Can you work these out from the model? Positions are in its coordinate system, mm. A direction names the side the tool comes from. Coordinates: 2 decimals unless noted, no trailing zeros. Write each loop counter-clockwise with the first axis right and the second up, starting at its lowest first coordinate (ties: lowest second). Pieces come first, ordered by that corner, then holes. Notation, with made-up numbers: (42.5, 34) -> (65.5, 34) arc R26 ccw to (65.5, 71) -> close; hole circle Ø10 at (54.5, 16). An arc over 180 degrees is marked (long way). Answer as CSV lines item,"result". Start each with the question number.
Autodesk Inventor part; units mm, degrees
ref_plane "YZ Plane" through (0, 0, 0) normal (1, 0, 0) x (0, 1, 0)
ref_plane "XZ Plane" through (0, 0, 0) normal (0, 1, 0) x (-1, 0, 0)
ref_plane "XY Plane" through (0, 0, 0) normal (0, 0, 1) x (1, 0, 0)
sketch "Sketch1" plane through (0, 0, 0) normal (0, 0, 1) x (1, 0, 0)
  line L0 (-19.313, 5.3077) -> (234.687, 5.3077)
  line L1 (234.687, 5.3077) -> (234.687, 0.3077)
  line L2 (234.687, 0.3077) -> (-19.313, 0.3077)
  line L3 (-19.313, 0.3077) -> (-19.313, 5.3077)
  line L4 (44.187, 5.3077) -> (44.187, 0.3077) construction
  line L5 (171.187, 5.3077) -> (171.187, 0.3077) construction
  line L6 (107.687, 5.3077) -> (107.687, 0.3077) construction
  point P0 (0, 0)
  dimension "d0" = 254
  dimension "d1" = 5
  dimension "d2" = 63.5
  dimension "d3" = 63.5
  dimension "d4" = 63.5
extrude "Extrusion1" add sketch "Sketch1" along normal blind 5
sketch "Sketch2" plane through (0, 0, 0) normal (0, 0, -1) x (-1, 0, 0)
  line L0 (19.313, 0.3077) -> (-234.687, 0.3077)
  arc A0 (-20.4966, 0.3077) -> (-14.937, 4.3077) centre (-20.4966, 6.1713) ccw
  arc A1 (-9.937, 4.3077) -> (-4.3774, 0.3077) centre (-4.3774, 6.1713) ccw
  line L1 (-14.937, 4.3077) -> (-9.937, 4.3077)
  line L2 (19.313, 0.3077) -> (-234.687, 0.3077)
  line L3 (-234.687, 5.3077) -> (19.313, 5.3077)
  arc A2 (-82.7042, 0.3077) -> (-78.437, 3.8077) centre (-82.7042, 4.659) ccw
  arc A3 (-73.437, 3.8077) -> (-69.1698, 0.3077) centre (-69.1698, 4.659) ccw
  line L4 (-78.437, 3.8077) -> (-73.437, 3.8077)
  arc A4 (-146.3937, 0.3077) -> (-141.937, 3.3077) centre (-146.3937, 5.1181) ccw
  arc A5 (-136.937, 3.3077) -> (-132.4803, 0.3077) centre (-132.4803, 5.1181) ccw
  line L5 (-141.937, 3.3077) -> (-136.937, 3.3077)
  arc A6 (-215.504, 0.3077) -> (-207.937, 4.3077) centre (-215.504, 9.4651) ccw
  arc A7 (-197.937, 4.3077) -> (-190.37, 0.3077) centre (-190.37, 9.4651) ccw
  line L6 (-207.937, 4.3077) -> (-197.937, 4.3077)
  line L7 (19.313, 5.3077) -> (19.313, 0.3077)
  point P0 (0, 0)
  point P1 (19.313, 2.8077)
  point P2 (-12.437, 4.3077)
  point P3 (-75.937, 3.8077)
  point P4 (-139.437, 3.3077)
  point P5 (-202.937, 4.3077)
  point P6 (-82.7042, 0.3077)
  point P7 (-69.1698, 0.3077)
  point P8 (-146.3937, 0.3077)
  point P9 (-132.4803, 0.3077)
  point P10 (-215.504, 0.3077)
  point P11 (-190.37, 0.3077)
  dimension "d7" = 1
  dimension "d8" = 1.5
  dimension "d9" = 2
  dimension "d10" = 1
  dimension "d11" = 5
  dimension "d12" = 10
  dimension "d14" = 31.75
  dimension "d15" = 63.5
  dimension "d16" = 63.5
  dimension "d17" = 63.5
extrude "Extrusion2" cut sketch "Sketch2" against normal through all
properties part number "Hingetest"
Q1. Imagine slicing it at B-B (y = 1.5). Write out the boundary of the cut face in (x, z), then the cut area to 3 significant figures.
Q2. Imagine slicing it at A-A (z = 2.95). Write out the boundary of the cut face in (x, y).
Q3. I need wall thicknesses on L1, parallel to X at y = 1.15, z = 0.8; L2, parallel to X at y = 2.7, z = 4.4; L3, parallel to Y at x = 205.5, z = 3.9. Which ranges of each line are inside material? Lowest first, please.
Q4. If we mould it in two halves opening along X, with no side actions, what happens to faces 1 (the face through (106, 3, 0)), 2 (the face through (-19.313, 3, 2)), 3 (the face through (79.977, 1.268, 2.465))? For each: released by +X, released by -X, zero draft, split by the parting line, or undercut.
Q5. For pin 1 (2.5 mm diameter, centred on x = 201, z = 3, fed in from -Y), with a flat end and sliding along its axis, tell me the tip position at first contact or that it passes through.
Q6. Which directions (+Z, -Z, +X, -X, +Y, -Y) give clear straight access to the entire face, cutting with the end or side of a thin tool? Please do faces 4 (the face through (203, 4.308, 2)), 5 (the face through (-7, 0.308, 2)).
Entries:
1,outline,"(-19.31, 0) -> (7.92, 0) -> (7.92, 5) -> (-19.31, 5) -> close; (16.95, 0) -> (72.16, 0) -> (72.16, 5) -> (16.95, 5) -> close; (79.71, 0) -> (135.65, 0) -> (135.65, 5) -> (79.71, 5) -> close; (143.22, 0) -> (194.89, 0) -> (194.89, 5) -> (143.22, 5) -> close; (210.99, 0) -> (234.69, 0) -> (234.69, 5) -> (210.99, 5) -> close"
1,area,"1,070 mm2"
2,outline,"(-19.31, 0.31) -> (4.38, 0.31) arc R5.86 ccw to (9.94, 4.31) -> (14.94, 4.31) arc R5.86 ccw to (20.5, 0.31) -> (69.17, 0.31) arc R4.35 ccw to (73.44, 3.81) -> (78.44, 3.81) arc R4.35 ccw to (82.7, 0.31) -> (132.48, 0.31) arc R4.81 ccw to (136.94, 3.31) -> (141.94, 3.31) arc R4.81 ccw to (146.39, 0.31) -> (190.37, 0.31) arc R9.16 ccw to (197.94, 4.31) -> (207.94, 4.31) arc R9.16 ccw to (215.5, 0.31) -> (234.69, 0.31) -> (234.69, 5.31) -> (-19.31, 5.31) -> close"
3,L1,"-19.31 to 7.41, 17.47 to 71.74, 80.13 to 135.2, 143.67 to 194.21, 211.67 to 234.69"
3,L2,"-19.31 to 9.1, 15.77 to 73.06, 78.82 to 136.64, 142.24 to 196.54, 209.33 to 234.69"
3,L3,"4.31 to 5.31"
4,face 1,"zero draft"
4,face 2,"released by -X"
4,face 3,"undercut"
5,pin 1,"y = 4.31"
6,face 4,"+Z, -Z, -Y"
6,face 5,"+Z, -Z, +X, -X, -Y"
